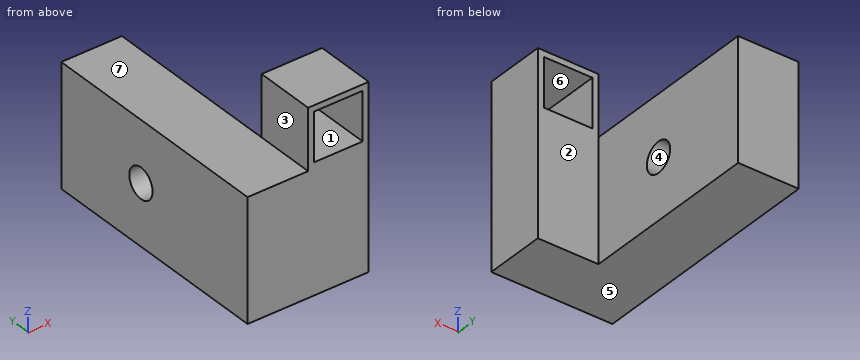
Autodesk Inventor part; units mm, degrees
ref_plane "YZ Plane" through (0, 0, 0) normal (1, 0, 0) x (0, 1, 0)
ref_plane "XZ Plane" through (0, 0, 0) normal (0, 1, 0) x (-1, 0, 0)
ref_plane "XY Plane" through (0, 0, 0) normal (0, 0, 1) x (1, 0, 0)
sketch "Sketch1" plane through (0, 0, 0) normal (0, 1, 0) x (-1, 0, 0)
  line L0 (25.4, 231.775) -> (25.4, 257.175)
  line L1 (25.4, 257.175) -> (0, 257.175)
  line L2 (0, 231.775) -> (0, 257.175)
  line L3 (25.4, 231.775) -> (0, 231.775)
  line L4 (2.54, 234.315) -> (2.54, 254.635)
  line L5 (2.54, 254.635) -> (22.86, 254.635)
  line L6 (22.86, 254.635) -> (22.86, 234.315)
  line L7 (22.86, 234.315) -> (2.54, 234.315)
  line L8 (25.4, 231.775) -> (0, 231.775)
  line L9 (0, 231.775) -> (0, 180.975)
  line L10 (0, 180.975) -> (25.4, 180.975)
  line L11 (25.4, 180.975) -> (25.4, 231.775)
  line L12 (25.4, 231.775) -> (25.4, 257.175)
  line L13 (25.4, 257.175) -> (0, 257.175)
  line L14 (0, 231.775) -> (0, 257.175)
  line L15 (25.4, 231.775) -> (0, 231.775)
  line L16 (2.54, 234.315) -> (2.54, 254.635)
  line L17 (2.54, 254.635) -> (22.86, 254.635)
  line L18 (22.86, 254.635) -> (22.86, 234.315)
  line L19 (22.86, 234.315) -> (2.54, 234.315)
  line L20 (25.4, 231.775) -> (0, 231.775)
  line L21 (0, 231.775) -> (0, 180.975)
  line L22 (0, 180.975) -> (25.4, 180.975)
  line L23 (25.4, 180.975) -> (25.4, 231.775)
  point P0 (0, 0)
  dimension "d0" = 50.8
  dimension "d1" = 50.8
extrude "Extrusion1" add sketch "Sketch1" along normal blind 25.4
sketch "Sketch2" plane through (0, 0, 0) normal (0, -1, 0) x (1, 0, 0)
  line L0 (-25.4, 180.975) -> (-25.4, 257.175)
  line L1 (-25.4, 180.975) -> (-50.8, 180.975)
  line L2 (-50.8, 180.975) -> (-50.8, 231.775)
  line L3 (-50.8, 231.775) -> (-25.4, 231.775)
  line L4 (-25.4, 231.775) -> (-25.4, 180.975)
  point P0 (0, 0)
  dimension "d4" = 25.4
  dimension "d5" = 50.8
extrude "Extrusion2" add sketch "Sketch2" against normal blind 101.6
sketch "Sketch5" plane through (-50.8, 0, 180.975) normal (-1, 0, 0) x (0, 0, 1)
  circle A0 centre (25.4, 19.05) radius 6.35 construction
  line L0 (25.4, 19.05) -> (25.4, 58.166) construction
  circle A1 centre (25.4, 58.166) radius 6.35
  point P0 (-180.975, 0)
  dimension "d10" = 39.116
  dimension "d11" = 12.7
extrude "Extrusion4" cut sketch "Sketch5" against normal blind 25.4
properties part number "intakee mount"
Input: part model. Units: mm. Frame: model coordinates. Face numbers are marked on the shaded views. A direction names the side the tool comes from. Give positions to 0.01 mm unless a question says otherwise; leave off trailing zeros. Order: outer loops, then holes, each group sorted by start corner. A loop starts at its lowest first (then second) coordinate and runs counter-clockwise, first axis right, second up.
Q1. Section B-B on z = 242.5. Output: boundary loops of the cut face in (x, y), and give its area (3 significant figures).
Checked values:
outline: (-25.4, 0) - (-22.86, 0) - (-22.86, 25.4) - (-25.4, 25.4) - close; (-2.54, 0) - (0, 0) - (0, 25.4) - (-2.54, 25.4) - close
area: 129 mm2
Q2. Section C-C on y = 13.5. Output: boundary loops of the cut face in (x, z) (3 decimals).
Checked values:
outline: (-50.8, 180.975) - (0, 180.975) - (0, 257.175) - (-25.4, 257.175) - (-25.4, 231.775) - (-50.8, 231.775) - close; hole (-22.86, 234.315) - (-2.54, 234.315) - (-2.54, 254.635) - (-22.86, 254.635) - close
Q3. Section D-D on z = 189. Output: boundary loops of the cut face in (x, y), and give its area (3 significant figures).
Checked values:
outline: (-50.8, 0) - (0, 0) - (0, 25.4) - (-25.4, 25.4) - (-25.4, 101.6) - (-50.8, 101.6) - close
area: 3,230 mm2
Q4. Set-up query: the marked faces 1, 2, 3 and 4. Return all of +Z, -Z, +X, -X, +Y, -Y with unobstructed straight access to the full face (end or side cutting, diameter ignored); none if empty.
Checked values:
face 1: +Y, -Y
face 2: +Z, -Z, +X, +Y
face 3: +Z, -X, +Y, -Y
face 4: +X, -X
Q5. Section A-A on x = -19.5. Output: boundary loops of the cut face in (y, z) (3 decimals), and give its area (3 significant figures).
Checked values:
outline: (0, 180.975) - (25.4, 180.975) - (25.4, 234.315) - (0, 234.315) - close; (0, 254.635) - (25.4, 254.635) - (25.4, 257.175) - (0, 257.175) - close
area: 1,420 mm2
Q6. Ray query, probe 1 along Z at (x, y) = (-19, 12) (3 decimals); probe 2 along Y at (x, z) = (-22.5, 210); probe 3 along X at (y, z) = (37, 190). Return the intervals inside material, ascending.
Checked values:
probe 1: z = 180.975 to 234.315, 254.635 to 257.175
probe 2: y = 0 to 25.4
probe 3: x = -50.8 to -25.4
Q7. Contact query for flat-ended pins moving along their axis: pin 1 Ø16.5 at (y, z) = (8.5, 244) entering from -X; pin 2 Ø8 at (x, z) = (-8, 199.5) entering from +Y; pin 3 Ø20.5 at (x, y) = (-37, 34.5) entering from +Z (3 decimals). Output: stop coordinate, or through.
Checked values:
pin 1: stops at x = -25.4
pin 2: stops at y = 25.4
pin 3: stops at z = 231.775
Q8. Draft query along Z for the marked faces 5, 6 and 7. Return one class per face: +Z half, -Z half, draft (parallel to the pull), parting line (faces both ways), or undercut.
Checked values:
face 5: -Z half
face 6: undercut
face 7: +Z half
